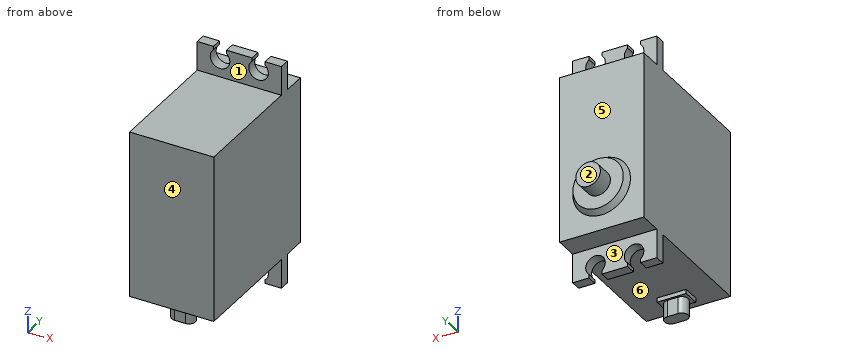
from build123d import *

# Parameters (mm, degrees)
BOSS_EXTRU_1_DEPTH      = 20.2
ESQUISSE2_R             = 2.35
ENL_V_MAT_EXTRU_1_DEPTH = 60.922366442
ESQUISSE8_W             = 3.1
ESQUISSE8_H             = 3.49339615
ENL_V_MAT_EXTRU_2_DEPTH = 10
ESQUISSE3_R             = 2.95
BOSS_EXTRU_2_DEPTH      = 5.7
ESQUISSE5_R             = 6.9
BOSS_EXTRU_4_DEPTH      = 1.5
BOSS_EXTRU_4_TAPER      = 30
ESQUISSE6_W             = 7
ESQUISSE6_H             = 4
BOSS_EXTRU_5_DEPTH      = 1
BOSS_EXTRU_6_DEPTH      = 4


with BuildPart() as part:
    # Esquisse1 → Boss.-Extru.1 (new body)
    with BuildSketch(Plane(origin=(0, 0, 0), x_dir=(0, 0, -1), z_dir=(1, 0, 0))):
        Polygon((0, 0), (40.2, 0), (40.2, 28.4), (47.2, 28.4), (47.2, 30.9), (40.2, 30.9), (40.2, 36.4), (0, 36.4), (0, 30.9), (-7, 30.9), (-7, 28.4), (0, 28.4), align=None)
    extrude(amount=BOSS_EXTRU_1_DEPTH)

    # Esquisse2 → Enlèv. mat.-Extru.1 (cut, through all)
    with BuildSketch(Plane(origin=(0, 30.9, 0), x_dir=(1, 0, 0), z_dir=(0, 1, 0))):
        with Locations(Location((5.475, 44.6, 0), (0, 0, 270))):
            Circle(ESQUISSE2_R)
        with Locations(Location((14.725, 44.6, 0), (0, 0, 270))):
            Circle(ESQUISSE2_R)
        with Locations(Location((14.725, -4.4, 0), (0, 0, 270))):
            Circle(ESQUISSE2_R)
        with Locations(Location((5.475, -4.4, 0), (0, 0, 270))):
            Circle(ESQUISSE2_R)
    extrude(amount=-ENL_V_MAT_EXTRU_1_DEPTH, mode=Mode.SUBTRACT)

    # Esquisse8 → Enlèv. mat.-Extru.2 (cut)
    with BuildSketch(Plane(origin=(0, 30.9, 0), x_dir=(1, 0, 0), z_dir=(0, 1, 0))):
        with Locations((5.475, 46.933629306)):
            Rectangle(ESQUISSE8_W, ESQUISSE8_H)
        with Locations((14.725, 46.933629306)):
            Rectangle(ESQUISSE8_W, ESQUISSE8_H)
        with Locations((14.725, -6.733629306)):
            Rectangle(ESQUISSE8_W, ESQUISSE8_H)
        with Locations((5.475, -6.733629306)):
            Rectangle(ESQUISSE8_W, ESQUISSE8_H)
    extrude(amount=-ENL_V_MAT_EXTRU_2_DEPTH, mode=Mode.SUBTRACT)

    # Esquisse3 → Boss.-Extru.2 (add)
    with BuildSketch(Plane(origin=(0, 36.4, 0), x_dir=(1, 0, 0), z_dir=(0, 1, 0))):
        with Locations(Location((10.1, 29.7, 0), (0, 0, 90))):
            Circle(ESQUISSE3_R)
    extrude(amount=BOSS_EXTRU_2_DEPTH)

    # Esquisse5 → Boss.-Extru.4 (add)
    with BuildSketch(Plane(origin=(0, 36.4, 0), x_dir=(1, 0, 0), z_dir=(0, 1, 0))):
        with Locations((10.1, 29.7)):
            Circle(ESQUISSE5_R)
    extrude(amount=BOSS_EXTRU_4_DEPTH, taper=BOSS_EXTRU_4_TAPER)

    # Esquisse6 → Boss.-Extru.5 (add)
    with BuildSketch(Plane(origin=(0, 0, -40.2), x_dir=(-1, 0, 0), z_dir=(0, 0, -1))):
        with Locations((-10.1, 5)):
            Rectangle(ESQUISSE6_W, ESQUISSE6_H)
    extrude(amount=BOSS_EXTRU_5_DEPTH)

    # Esquisse7 → Boss.-Extru.6 (add)
    with BuildSketch(Plane(origin=(0, 0, -41.2), x_dir=(-1, 0, 0), z_dir=(0, 0, -1))):
        with BuildLine():
            Line((-11.4, 6.55), (-8.8, 6.55))
            ThreePointArc((-8.8, 6.55), (-7.25, 5), (-8.8, 3.45))
            Line((-8.8, 3.45), (-11.4, 3.45))
            ThreePointArc((-11.4, 3.45), (-12.95, 5), (-11.4, 6.55))
        make_face()
    extrude(amount=BOSS_EXTRU_6_DEPTH)


solid = part.part
Source: CAD feature listing. Evaluate the final solid. Frame: model axes, mm. Face numbers are marked on the shaded views. A direction names the side the tool comes from. Round coordinates to 2 decimals unless told otherwise and drop trailing zeros. Loops run counter-clockwise (first coordinate to the right, second up) from the corner with the lowest first, then second, coordinate; pieces in that order, holes last. Notation, with made-up numbers: M 73,-22.75 L 98,-22.75 A4 ccw 98,-18.75 Z; hole C 86,7.25 d11. An arc over 180 degrees is marked long. Return JSON: item names as keys, results as strings. Group by question number.
1. Section query A-A on z = 4.4. Output: boundary loops of the cut face in (x, y) (3 decimals).
2. Material intervals for line 1 along X through (y, z) = (29.4, 4.4) (3 decimals); line 2 along Y through (x, z) = (8.75, -41.5); line 3 along Y through (x, z) = (18, -14), sorted ascending. Write a range as from..to.
3. Section query C-C on y = 20.5. Output: boundary loops of the cut face in (x, z), and give its area (3 significant figures).
4. Section query B-B on x = 1.5. Output: boundary loops of the cut face in (y, z), and give its area (3 significant figures).
5. Mould query, pull axis Y, two halves, no side actions, for the marked faces 4, 5 and 6. Classes: released by +Y, released by -Y, zero draft, split by the parting line, or undercut.
6. Pin query (flat end, axial travel): pin 1 (4.5 mm diameter, centred on x = 14, y = 35, fed in from -Z); pin 2 (2 mm diameter, centred on x = 14.5, z = -42.5, fed in from +Y); pin 3 (2 mm diameter, centred on y = 12.5, z = -15.5, fed in from -X); pin 4 (3 mm diameter, centred on x = 10.5, y = 5, fed in from -Z). Return the tip coordinate at first contact, or that it passes through.
7. Section query D-D on z = -21. Output: boundary loops of the cut face in (x, y).
8. Reachability of the marked faces 1, 2 and 3 from +Z, -Z, +X, -X, +Y, -Y: full face, straight path, thin tool, end or side. Return the list, or none.
Checks:
{
 "1": {"outline": "M 0,28.4 L 3.125,28.4 L 3.125,30.9 L 0,30.9 Z; M 7.825,28.4 L 12.375,28.4 L 12.375,30.9 L 7.825,30.9 Z; M 17.075,28.4 L 20.2,28.4 L 20.2,30.9 L 17.075,30.9 Z"},
 "2": {"line 1": "x = 0..3.125, 7.825..12.375, 17.075..20.2", "line 2": "y = 3.45..6.55, 28.4..30.9", "line 3": "y = 0..36.4"},
 "3": {"outline": "M 0,-40.2 L 20.2,-40.2 L 20.2,0 L 0,0 Z", "area": "812 mm²"},
 "4": {"outline": "M 0,-40.2 L 28.4,-40.2 L 28.4,-47.2 L 30.9,-47.2 L 30.9,-40.2 L 36.4,-40.2 L 36.4,0 L 30.9,0 L 30.9,7 L 28.4,7 L 28.4,0 L 0,0 Z", "area": "1,500 mm²"},
 "5": {"face 4": "released by -Y", "face 5": "released by +Y", "face 6": "undercut"},
 "6": {"pin 1": "stops at z = -40.2", "pin 2": "stops at y = 30.9", "pin 3": "stops at x = 0", "pin 4": "stops at z = -45.2"},
 "7": {"outline": "M 0,0 L 20.2,0 L 20.2,36.4 L 0,36.4 Z"},
 "8": {"face 1": "+Z, +X, -X, -Y", "face 2": "+Z, -Z, +X, -X, +Y", "face 3": "-Z, +X, -X, +Y"}
}
